Design review of the part built by this model. Coordinates are the model's own, in mm. A direction names the side the tool comes from. Give positions to 0.01 mm unless a question says otherwise; leave off trailing zeros. Loops run counter-clockwise (first coordinate to the right, second up) from the corner with the lowest first, then second, coordinate; pieces in that order, holes last. Notation, with made-up numbers: (22.5, 59) -> (81.5, 59) arc R16 ccw to (81.5, 85) -> close; hole circle Ø4 at (-22.75, -25). An arc over 180 degrees is marked (long way). Answer in a Markdown table with one row per item. Add a question column.
(1) For pin 1 (3 mm diameter, centred on x = 12.5, z = 8, fed in from +Y); pin 2 (6.5 mm diameter, centred on x = -47, y = 10.5, fed in from +Z); pin 3 (2 mm diameter, centred on x = 13.5, z = 2.5, fed in from -Y); pin 4 (2.5 mm diameter, centred on x = -46.5, y = 14.5, fed in from -Z), all flat-tipped, find the tip position at first contact; note any pin that passes through.
(2) Consider section A-A on x = -46. Write out the cut boundary in (y, z).
(3) Consider section B-B on z = -5.5. Write out the cut boundary in (x, y), then the cut area to 3 significant figures.
(4) Consider section D-D on y = 12.5. Write out the cut boundary in (x, z), then the cut area to 3 significant figures.
(5) Consider section C-C on x = 16.5. Write out the cut boundary in (y, z).
(6) For faces 1 (the flat face through (-42, 12, 0)), 2 (the flat face through (50, 3, 0)), 3 (the flat face through (-47, 11, 0.6)), 4 (the flat face through (-21, 4, -1.122)), list the 3-axis set-ups (+Z, -Z, +X, -X, +Y, -Y) from which the entire face can be reached by the end or side of a thin tool; tool diameter is ignored.
(7) Draft analysis for pull direction X (two halves, no side actions). For faces 5 (the flat face through (-46, 17, 0)), 6 (the flat face through (23, 4, -1.5)), 7 (the flat face through (-21.686, 4, 0)), 8 (the flat face through (-50, 5, 0)), state which applies: +X half, -X half, draft (parallel to the pull), parting line (faces both ways), or undercut.
(8) For line 1 (X direction, y = 4, z = 5.5); line 2 (Y direction, x = -26.5, z = 5); line 3 (X direction, y = 14.5, z = 0.75), list the stretches that pass through material, from the lowest coordinate up.
from build123d import *

# Parameters (mm, degrees)
SKETCH1_W           = 100
SKETCH1_H           = 20
BOSS_EXTRUDE1_DEPTH = 7
SKETCH2_W           = 8
SKETCH2_H           = 2
BOSS_EXTRUDE2_DEPTH = 10
SKETCH3_W           = 1.2
SKETCH3_H           = 8.2
CUT_EXTRUDE1_DEPTH  = 6.5
SKETCH4_R           = 1.5
CUT_EXTRUDE2_DEPTH  = 16.5
CUT_EXTRUDE3_DEPTH  = 16.5
CUT_EXTRUDE4_DEPTH  = 16.5


with BuildPart() as part:
    # Sketch1 → Boss-Extrude1 (new body)
    with BuildSketch(Plane(origin=(0, 0, 0), x_dir=(1, 0, 0), z_dir=(0, 1, 0))):
        Rectangle(SKETCH1_W, SKETCH1_H)
    extrude(amount=BOSS_EXTRUDE1_DEPTH)

    # Sketch2 → Boss-Extrude2 (add)
    with BuildSketch(Plane(origin=(0, 7, 0), x_dir=(1, 0, 0), z_dir=(0, 1, 0))):
        with Locations((-46, 0)):
            Rectangle(SKETCH2_W, SKETCH2_H)
    extrude(amount=BOSS_EXTRUDE2_DEPTH)

    # Sketch3 → Cut-Extrude1 (cut)
    with BuildSketch(Plane.ZY.offset(50)):
        with Locations((0, 11.1)):
            Rectangle(SKETCH3_W, SKETCH3_H)
    extrude(amount=-CUT_EXTRUDE1_DEPTH, mode=Mode.SUBTRACT)

    # Sketch4 → Cut-Extrude2 (cut)
    with BuildSketch(Plane(origin=(0, 7, 0), x_dir=(1, 0, 0), z_dir=(0, 1, 0))):
        with Locations(Location((-46, -5.5, 0), (0, 0, 270))):
            Circle(SKETCH4_R)
        with Locations(Location((-46, 5.5, 0), (0, 0, 270))):
            Circle(SKETCH4_R)
    extrude(amount=-CUT_EXTRUDE2_DEPTH, mode=Mode.SUBTRACT)

    # Sketch5 → Cut-Extrude3 (cut)
    with BuildSketch(Plane(origin=(0, 7, 0), x_dir=(1, 0, 0), z_dir=(0, 1, 0))):
        with BuildLine():
            Line((4, 1.5), (42.104534382, 1.5))
            ThreePointArc((42.104534382, 1.5), (43.604534382, 0), (42.104534382, -1.5))
            Line((42.104534382, -1.5), (4, -1.5))
            ThreePointArc((4, -1.5), (2.5, 0), (4, 1.5))
        make_face()
    extrude(amount=-CUT_EXTRUDE3_DEPTH, mode=Mode.SUBTRACT)

    # Sketch6 → Cut-Extrude4 (cut)
    with BuildSketch(Plane(origin=(0, 7, 0), x_dir=(1, 0, 0), z_dir=(0, 1, 0))):
        with BuildLine():
            Line((-38.090566617, 1.691624874), (-36.136720463, 1.691624874))
            Line((-36.136720463, 1.691624874), (-36.136720463, -0.374160382))
            add(Edge.make_bspline(
                [(-36.136720463, -0.374160382), (-36.136222921, -0.395596016), (-36.135259527, -0.437102045), (-36.128176252, -0.496659376), (-36.117267464, -0.551720243), (-36.099494327, -0.601255913), (-36.079050673, -0.647053262), (-36.052579871, -0.687323798), (-36.021884122, -0.723028206), (-35.985294073, -0.753165432), (-35.943444242, -0.779987134), (-35.896520116, -0.806221032), (-35.842987125, -0.830109847), (-35.783305155, -0.852165702), (-35.717831736, -0.873864468), (-35.646135273, -0.894146598), (-35.56817414, -0.912378535), (-35.484446285, -0.929627894), (-35.395305953, -0.944570047), (-35.30137293, -0.958050388), (-35.202951382, -0.969319491), (-35.100128875, -0.979013349), (-34.99279273, -0.985787257), (-34.881047838, -0.990848531), (-34.764636845, -0.99407686), (-34.685542294, -0.99463124), (-34.645259125, -0.994913587)],
                knots=[0, 0, 0, 0, 0.856800499, 1.659031242, 2.395514242, 3.095174505, 3.758838491, 4.395989299, 5.014775861, 5.634490662, 6.283374298, 7.000480573, 7.781977864, 8.624273548, 9.543693618, 10.539207642, 11.602158877, 12.744227547, 13.956608171, 15.215308399, 16.537999948, 17.91707144, 19.344177482, 20.837586847, 22.389370407, 24, 24, 24, 24], degree=3))
            add(Edge.make_bspline(
                [(-34.645259125, -0.994913587), (-34.602644304, -0.994619773), (-34.518887139, -0.994042296), (-34.395467432, -0.990967311), (-34.276493626, -0.985329628), (-34.162218877, -0.976931814), (-34.05233768, -0.966910998), (-33.947109184, -0.954375876), (-33.846232554, -0.938820672), (-33.750290053, -0.922073681), (-33.660190511, -0.902955674), (-33.576791977, -0.882732471), (-33.500569827, -0.861280306), (-33.431693571, -0.838617434), (-33.370513532, -0.814205685), (-33.315903174, -0.789823701), (-33.268859004, -0.763186911), (-33.228027111, -0.734837962), (-33.193111029, -0.702177186), (-33.163728858, -0.66337951), (-33.138706328, -0.618201192), (-33.118757714, -0.566526559), (-33.102800885, -0.508586363), (-33.091478933, -0.444294518), (-33.085510067, -0.373424974), (-33.084409099, -0.324137339), (-33.083835848, -0.298474285)],
                knots=[0, 0, 0, 0, 1.588209429, 3.121541213, 4.600766171, 6.026677194, 7.391541964, 8.712617744, 9.975319141, 11.1950937, 12.341822282, 13.407306122, 14.392766533, 15.292249026, 16.108021068, 16.846936864, 17.51923127, 18.119926431, 18.695626892, 19.292987148, 19.926115191, 20.614241253, 21.352269412, 22.162859459, 23.043438806, 24, 24, 24, 24], degree=3))
            Line((-33.083835848, -0.298474285), (-33.083835848, 1.691624874))
            Line((-33.083835848, 1.691624874), (-31.129989694, 1.691624874))
            Line((-31.129989694, 1.691624874), (-31.129989694, -0.202435623))
            add(Edge.make_bspline(
                [(-31.129989694, -0.202435623), (-31.130396555, -0.240823825), (-31.131179852, -0.314729458), (-31.139375273, -0.420958153), (-31.153266871, -0.518056089), (-31.172113358, -0.60591195), (-31.195776106, -0.685102071), (-31.2265614, -0.75468246), (-31.261807566, -0.815796798), (-31.304224039, -0.868565412), (-31.35433564, -0.915957753), (-31.413244095, -0.961750023), (-31.482378453, -1.006475356), (-31.560729801, -1.051863818), (-31.649567417, -1.096031718), (-31.747973897, -1.140446708), (-31.856395889, -1.184349919), (-31.973869243, -1.226902741), (-32.098340547, -1.26900542), (-32.228765844, -1.30740489), (-32.363828076, -1.343760755), (-32.503536352, -1.37752487), (-32.648066029, -1.407754368), (-32.797051714, -1.436069214), (-32.950903144, -1.460434965), (-33.109645942, -1.483126236), (-33.274098084, -1.501657516), (-33.444488933, -1.519283924), (-33.621592617, -1.533001036), (-33.805232974, -1.544180789), (-33.995384773, -1.554126205), (-34.192171214, -1.560117111), (-34.395499456, -1.564098136), (-34.533317979, -1.564553974), (-34.603281962, -1.564785382)],
                knots=[0, 0, 0, 0, 0.891995564, 1.717285311, 2.473985171, 3.169784855, 3.80406141, 4.390865003, 4.934193818, 5.438959715, 5.958162933, 6.533752086, 7.170549563, 7.870280448, 8.637066367, 9.475009947, 10.378954102, 11.354689114, 12.378321379, 13.432112796, 14.513721255, 15.6286606, 16.771808402, 17.944919068, 19.152624798, 20.3914954, 21.671212985, 22.998319501, 24.372293643, 25.798941139, 27.273951603, 28.797175972, 30.374076868, 32, 32, 32, 32], degree=3))
            add(Edge.make_bspline(
                [(-34.603281962, -1.564785382), (-34.694874664, -1.564329464), (-34.875124498, -1.563432241), (-35.141015791, -1.555385336), (-35.398042018, -1.543673109), (-35.645950763, -1.52656085), (-35.884746849, -1.504366425), (-36.114450133, -1.477165199), (-36.335189293, -1.444656968), (-36.546015909, -1.408065912), (-36.74501405, -1.367761314), (-36.92986633, -1.323831929), (-37.100308606, -1.278213772), (-37.255996039, -1.230308582), (-37.396994074, -1.179518335), (-37.523325041, -1.126403766), (-37.634981713, -1.070496906), (-37.733587124, -1.012166957), (-37.819089301, -0.946207757), (-37.892334947, -0.870525317), (-37.954025458, -0.784041833), (-38.004293928, -0.687432955), (-38.043166993, -0.580459305), (-38.07089232, -0.463535136), (-38.087398684, -0.336257042), (-38.089486381, -0.248067484), (-38.090566617, -0.202435623)],
                knots=[0, 0, 0, 0, 1.595870397, 3.140592737, 4.634612613, 6.078715518, 7.46998073, 8.812936474, 10.108520143, 11.357136621, 12.540896352, 13.645651431, 14.667177183, 15.61474762, 16.482960095, 17.277467721, 18.001045958, 18.65737072, 19.270672542, 19.876756492, 20.485670631, 21.115189159, 21.768481852, 22.463746561, 23.205097451, 24, 24, 24, 24], degree=3))
            Line((-38.090566617, -0.202435623), (-38.090566617, 1.691624874))
        make_face()
        Polygon((-25.471976873, 1.691624874), (-19.854669181, 1.691624874), (-19.854669181, 1.121753079), (-21.68639995, 1.121753079), (-21.68639995, -1.483375126), (-23.640246104, -1.483375126), (-23.640246104, 1.121753079), (-25.471976873, 1.121753079), align=None)
        Polygon((-13.19938072, 1.691624874), (-11.300868099, 1.691624874), (-8.925342258, -0.522988507), (-6.539004117, 1.691624874), (-4.653211849, 1.691624874), (-2.921335848, -1.483375126), (-4.819848468, -1.483375126), (-5.913162771, 0.521988456), (-8.074350671, -1.483375126), (-9.786510127, -1.483375126), (-11.937521745, 0.521988456), (-13.03020003, -1.483375126), (-14.929348668, -1.483375126), align=None)
    extrude(amount=-CUT_EXTRUDE4_DEPTH, mode=Mode.SUBTRACT)


solid = part.part
Values follow:
| question | item | result |
|---|---|---|
| 1 | pin 1 | y = 7 |
| 1 | pin 2 | z = 1 |
| 1 | pin 3 | y = 0 |
| 1 | pin 4 | z = -1 |
| 2 | outline | (0, -10) -> (7, -10) -> (7, -7) -> (0, -7) -> close; (0, -4) -> (7, -4) -> (7, -1) -> (17, -1) -> (17, 1) -> (7, 1) -> (7, 4) -> (0, 4) -> close; (0, 7) -> (7, 7) -> (7, 10) -> (0, 10) -> close; hole (7, -0.6) -> (15.2, -0.6) -> (15.2, 0.6) -> (7, 0.6) -> close |
| 3 | outline | (-50, 0) -> (-47.5, 0) -> (-47.5, 7) -> (-50, 7) -> close; (-44.5, 0) -> (50, 0) -> (50, 7) -> (-44.5, 7) -> close |
| 3 | area | 679 mm2 |
| 4 | outline | (-50, -1) -> (-42, -1) -> (-42, 1) -> (-50, 1) -> (-50, 0.6) -> (-43.5, 0.6) -> (-43.5, -0.6) -> (-50, -0.6) -> close |
| 4 | area | 8.20 mm2 |
| 5 | outline | (0, -10) -> (7, -10) -> (7, -1.5) -> (0, -1.5) -> close; (0, 1.5) -> (7, 1.5) -> (7, 10) -> (0, 10) -> close |
| 6 | face 1 | +Z, -Z, +X, +Y |
| 6 | face 2 | +Z, -Z, +X, +Y, -Y |
| 6 | face 3 | -X |
| 6 | face 4 | +Y, -Y |
| 7 | face 5 | draft |
| 7 | face 6 | undercut |
| 7 | face 7 | undercut |
| 7 | face 8 | -X half |
| 8 | line 1 | -50 to -47.5, -44.5 to 50 |
| 8 | line 2 | 0 to 7 |
| 8 | line 3 | -50 to -42 |
